Design review of the part shown in the three views and the two pictorial views. Dimensions are in mm from the part's minimum x, y and z. A direction names the side the tool comes from. Coordinates: 2 decimals unless noted, no trailing zeros. Loops run counter-clockwise (first coordinate to the right, second up) from the corner with the lowest first, then second, coordinate; pieces in that order, holes last. Notation, with made-up numbers: (74.5, -37.5) -> (104.5, -37.5) arc R29 ccw to (104.5, -14.5) -> close; hole circle Ø9 at (20, 55.5). An arc over 180 degrees is marked (long way). Answer in a Markdown table with one row per item.
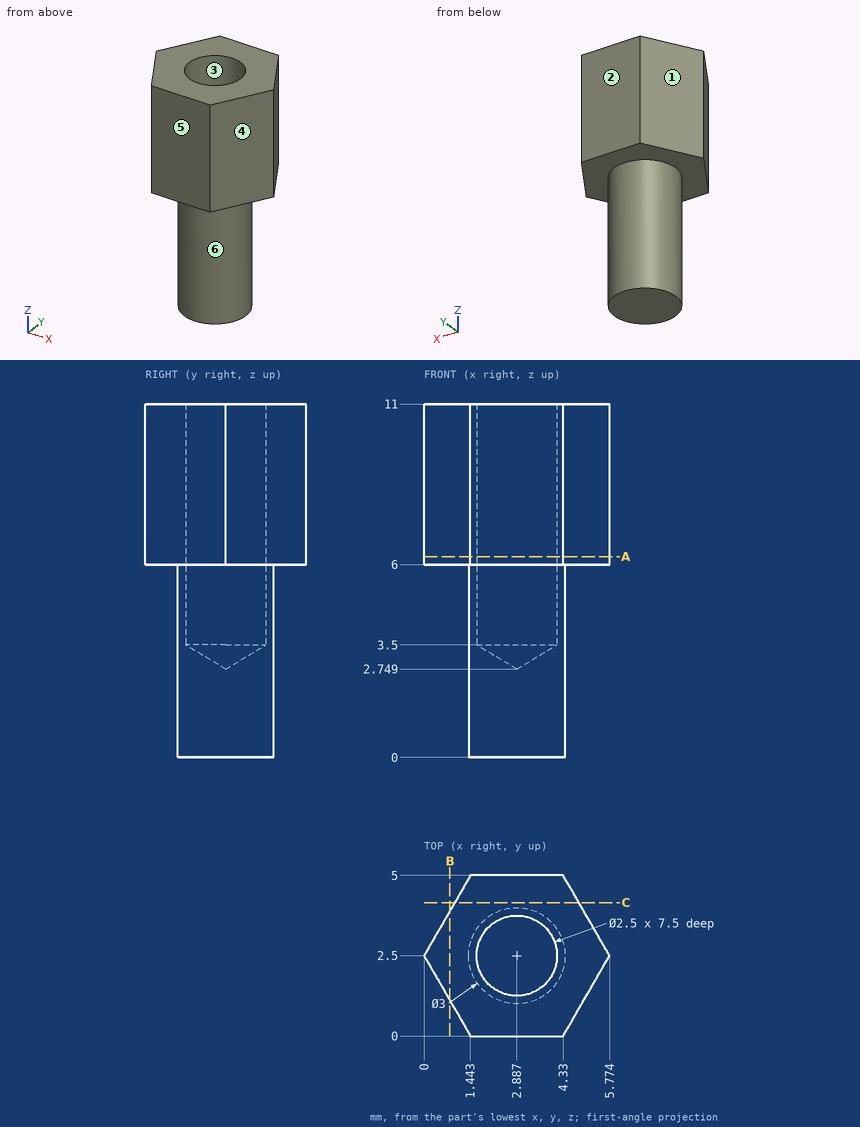
Item 1: For the marked faces 5 and 6, list the 3-axis set-ups (+Z, -Z, +X, -X, +Y, -Y) from which the entire face can be reached by the end or side of a thin tool; tool diameter is ignored.
Worked answers:
| item | result |
|---|---|
| face 5 | +Z, -Z, +X, -X, -Y |
| face 6 | -Z |
Item 2: The part is to be moulded in two halves that separate along X. For the marked faces 1, 2, 3 and 4, say which applies: +X half, -X half, draft (parallel to the pull), parting line (faces both ways), or undercut.
Worked answers:
| item | result |
|---|---|
| face 1 | -X half |
| face 2 | draft |
| face 3 | undercut |
| face 4 | +X half |
Item 3: Take a section at B-B, the plane x = 0.8. State the section outline as (y, z) points (1 decimal).
Worked answers:
| item | result |
|---|---|
| outline | (1.1, 6) -> (3.9, 6) -> (3.9, 11) -> (1.1, 11) -> close |
Item 4: For L1, parallel to Y at x = 2.95, z = 7.5; L2, parallel to Z at x = 0.7, y = 2.15; L3, parallel to X at y = 2.55, z = 7.5 (1 decimal), list the stretches that pass through material, from the lowest coordinate up.
Worked answers:
| item | result |
|---|---|
| L1 | 0 to 1.25, 3.75 to 5 |
| L2 | 6 to 11 |
| L3 | 0 to 1.6, 4.1 to 5.7 |
Item 5: Take a section at C-C, the plane y = 4.15. State the section outline as (x, z) points.
Worked answers:
| item | result |
|---|---|
| outline | (0.95, 6) -> (4.82, 6) -> (4.82, 11) -> (0.95, 11) -> close |
Item 6: Take a section at A-A, the plane z = 6.25. State the section outline as (x, y) points.
Worked answers:
| item | result |
|---|---|
| outline | (0, 2.5) -> (1.44, 0) -> (4.33, 0) -> (5.77, 2.5) -> (4.33, 5) -> (1.44, 5) -> close; hole circle Ø2.5 at (2.89, 2.5) |
Item 7: Insertion check: pin 1 (1 mm diameter, centred on y = 1, z = 9.5, fed in from +X) (1 decimal); pin 2 (1 mm diameter, centred on x = 2.5, y = 0.5, fed in from -Z). Each pin has a flat end and moves straight along its axis. Give the tip position at first contact, or say it passes through.
Worked answers:
| item | result |
|---|---|
| pin 1 | x = 5.2 |
| pin 2 | z = 6 |
